For this review, use the dimensioned drawing (mm, ordinates from the lowest corner) and the shaded views. Give positions to 0.01 mm unless a question says otherwise; leave off trailing zeros. Order: outer loops, then holes, each group sorted by start corner. A loop starts at its lowest first (then second) coordinate and runs counter-clockwise, first axis right, second up. Notation, with made-up numbers: M 41.5,21.5 L 66.5,21.5 A34 cw 66.5,51.5 Z; hole C 89,-25 d3. An arc over 180 degrees is marked long. Answer as CSV lines item,"result". Start each with the question number.
1. We need section B-B, the plane x = 20. Give the boundary of the cut face in (y, z), and give its area (3 significant figures).
2. Clearance check with flat-ended pins moving along their axes: P1, Ø3, axis at x = 13.5, z = 15.5, coming from the -Y side; P2, Ø1.5, axis at x = 35.5, y = 21, coming from the -Z side; P3, Ø10.5, axis at x = 20, z = 30, coming from the -Y side; P4, Ø8, axis at x = 18, y = 26.5, coming from the +Z side. State where each tip first meets the part, or that it passes through.
3. We need section A-A, the plane y = 20. Give the boundary of the cut face in (x, z).
4. We need section C-C, the plane z = 10.5. Give the boundary of the cut face in (x, y).
5. For line 1 along Y through (x, z) = (20, 10.5); line 2 along Z through (x, y) = (20, 36); line 3 along Z through (x, y) = (35, 33), list the stretches that pass through material, from the lowest coordinate up.
6. Mouldability with a two-part tool opening along X and no side actions: class the marked faces 1, 2 and 3 as pulls with the +X half, pulls with the -X half, needs draft (parallel to the pull), parting line crosses it, or undercut.
7. We need section D-D, the plane y = 8. Give the boundary of the cut face in (x, z), and give its area (3 significant figures).
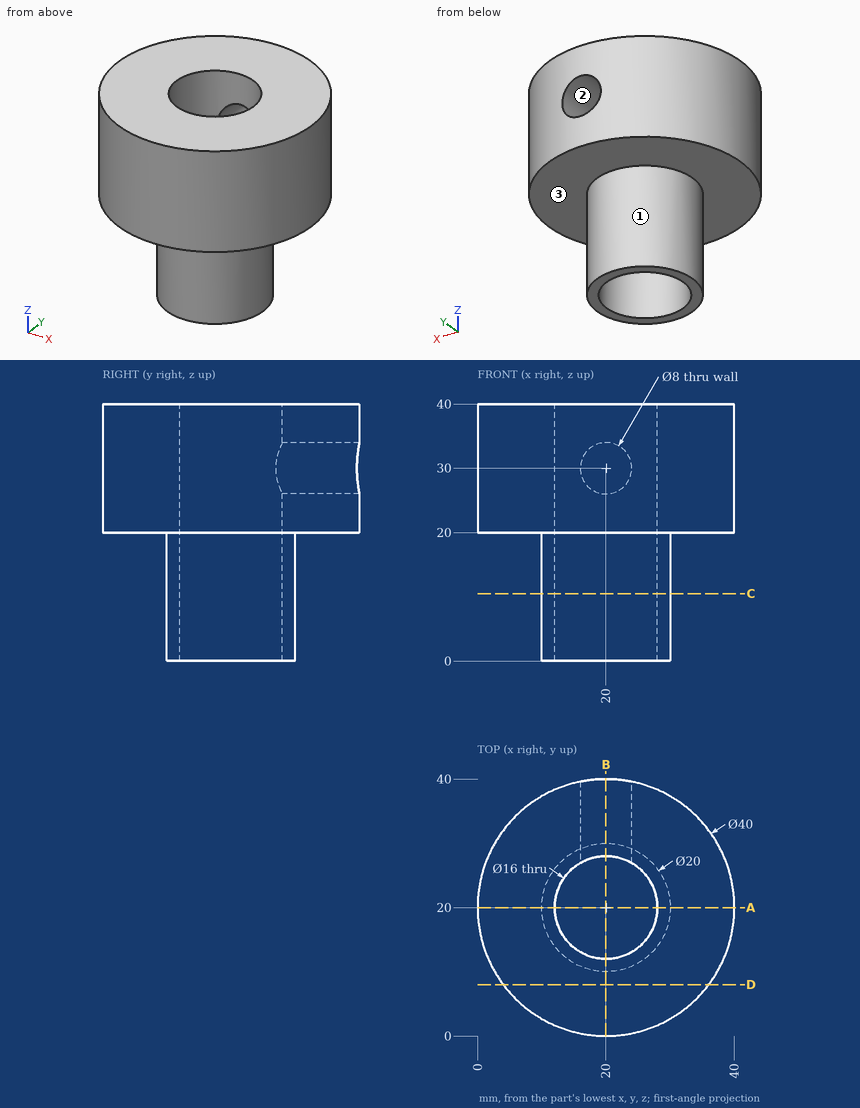
Result set:
1,outline,"M 0,20 L 10,20 L 10,0 L 12,0 L 12,40 L 0,40 Z; M 28,0 L 30,0 L 30,20 L 40,20 L 40,26 L 28,26 Z; M 28,34 L 40,34 L 40,40 L 28,40 Z"
1,area,"464 mm2"
2,P1,"y = 11.34"
2,P2,"z = 20"
2,P3,"y = 0"
2,P4,"z = 40"
3,outline,"M 0,20 L 10,20 L 10,0 L 12,0 L 12,40 L 0,40 Z; M 28,0 L 30,0 L 30,20 L 40,20 L 40,40 L 28,40 Z"
4,outline,"C 20,20 d20; hole C 20,20 d16"
5,line 1,"10 to 12, 28 to 30"
5,line 2,"20 to 26, 34 to 40"
5,line 3,"20 to 40"
6,face 1,"parting line crosses it"
6,face 2,"undercut"
6,face 3,"needs draft"
7,outline,"M 4,20 L 36,20 L 36,40 L 4,40 Z"
7,area,"640 mm2"
